For this review, take the finished solid that the model builds, in its own axes (mm). A direction names the side the tool comes from. Coordinates: 2 decimals unless noted, no trailing zeros. Order: outer loops, then holes, each group sorted by start corner. A loop starts at its lowest first (then second) coordinate and runs counter-clockwise, first axis right, second up. Notation, with made-up numbers: (77, 35) - (102, 35) arc R20 ccw to (102, 40) - close; hole circle Ø7 at (57, -4.75). An arc over 180 degrees is marked (long way). One line per item, written item: value. Start each with the question number.
(1) Mouldability with a two-part tool opening along Z and no side actions: class faces 1 (the cylindrical face through (-2.215, 1.014, -28.199)), 2 (the cylindrical face through (-2.199, 1.014, 2.215)), 3 (the cylindrical face through (7.805, 1.014, -27.487)) as released by +Z, released by -Z, zero draft, split by the parting line, or undercut.
(2) Consider section A-A on z = -21. Write out the cut boundary in (x, y), then the cut area to 3 significant figures.
(3) Consider section C-C on x = 0. Write out the cut boundary in (y, z), then the cut area to 3 significant figures.
(4) Consider section B-B on x = 4. Write out the cut boundary in (y, z), then the cut area to 3 significant figures.
(5) Consider section D-D on y = 0.4. Write out the cut boundary in (x, z).
(6) Clearance check with flat-ended pins moving along their axes: pin 1 (3.5 mm diameter, centred on x = 8, z = 0, fed in from +Y); pin 2 (1.8 mm diameter, centred on x = 0, z = -26, fed in from +Y). State where each tip first meets the part, or that it passes through.
(7) For faces 4 (the cylindrical face through (5.715, 1.014, -23.699)), 5 (the cylindrical face through (10.199, 1.014, 2.215)), list the 3-axis set-ups (+Z, -Z, +X, -X, +Y, -Y) from which the entire face can be reached by the end or side of a thin tool; tool diameter is ignored.
(8) To check wall thickness, follow line 1 along Z through (x, y) = (8, 0.8); line 2 along X through (y, z) = (1.4, -26); line 3 along X through (y, z) = (1.95, -8). State the ranges of each line that lie inside material, in increasing order.
```python
from build123d import *

# Parameters (mm, degrees)
SKETCH1_R           = 1.4
BOSS_EXTRUDE2_DEPTH = 5.5
FILLET2_R           = 1
SKETCH2_R           = 1.5
CUT_EXTRUDE1_DEPTH  = 10
SKETCH3_R           = 36.045042524
CUT_EXTRUDE2_DEPTH  = 0.5
SKETCH4_R           = 41.346922652
CUT_EXTRUDE3_DEPTH  = 1
SKETCH5_R           = 64.87410788
CUT_EXTRUDE4_DEPTH  = 2


with BuildPart() as part:
    # Sketch1 → Boss-Extrude2 (new body)
    with BuildSketch(Plane(origin=(0, 0, 0), x_dir=(1, 0, 0), z_dir=(0, 1, 0))):
        Polygon((4, -2.5), (-2.5, -2.5), (-2.5, 28.5), (10.5, 28.5), (10.5, -2.5), align=None)
        with Locations((8, 26)):
            Circle(SKETCH1_R, mode=Mode.SUBTRACT)
        with Locations((0, 26)):
            Circle(SKETCH1_R, mode=Mode.SUBTRACT)
        with Locations((8, 0)):
            Circle(SKETCH1_R, mode=Mode.SUBTRACT)
        Circle(SKETCH1_R, mode=Mode.SUBTRACT)
        Polygon((4, 2), (2, 2), (2, 24), (6, 24), (6, 2), align=None, mode=Mode.SUBTRACT)
    extrude(amount=BOSS_EXTRUDE2_DEPTH)

    # Fillet2
    fillet2_edges = [part.edges().sort_by_distance(p)[0] for p in [
        (6, 2.75, -24),
        (2, 2.75, -24),
        (2, 2.75, -2),
        (6, 2.75, -2),
        (-2.5, 2.75, 2.5),
        (-2.5, 2.75, -28.5),
        (10.5, 2.75, -28.5),
        (10.5, 2.75, 2.5),
    ]]
    fillet(fillet2_edges, radius=FILLET2_R)

    # Sketch2 → Cut-Extrude1 (cut)
    with BuildSketch(Plane(origin=(0, 5.5, 0), x_dir=(1, 0, 0), z_dir=(0, 1, 0))):
        with Locations((0, 26)):
            Circle(SKETCH2_R)
        with Locations((8, 26)):
            Circle(SKETCH2_R)
        with Locations((8, 0)):
            Circle(SKETCH2_R)
        Circle(SKETCH2_R)
    extrude(amount=-CUT_EXTRUDE1_DEPTH, mode=Mode.SUBTRACT)

    # Sketch3 → Cut-Extrude2 (cut)
    with BuildSketch(Plane(origin=(0, 5.5, 0), x_dir=(1, 0, 0), z_dir=(0, 1, 0))):
        Circle(SKETCH3_R)
    extrude(amount=-CUT_EXTRUDE2_DEPTH, mode=Mode.SUBTRACT)

    # Sketch4 → Cut-Extrude3 (cut)
    with BuildSketch(Plane(origin=(0, 5, 0), x_dir=(1, 0, 0), z_dir=(0, 1, 0))):
        Circle(SKETCH4_R)
    extrude(amount=-CUT_EXTRUDE3_DEPTH, mode=Mode.SUBTRACT)

    # Sketch5 → Cut-Extrude4 (cut)
    with BuildSketch(Plane(origin=(0, 4, 0), x_dir=(1, 0, 0), z_dir=(0, 1, 0))):
        Circle(SKETCH5_R)
    extrude(amount=-CUT_EXTRUDE4_DEPTH, mode=Mode.SUBTRACT)


solid = part.part
```
Geometry check:
1. face 1: released by -Z
1. face 2: released by +Z
1. face 3: undercut
2. outline: (-2.5, 0) - (2, 0) - (2, 2) - (-2.5, 2) - close; (6, 0) - (10.5, 0) - (10.5, 2) - (6, 2) - close
2. area: 18.0 mm^2
3. outline: (0, -28.5) - (2, -28.5) - (2, -27.5) - (0, -27.5) - close; (0, -24.5) - (2, -24.5) - (2, -1.5) - (0, -1.5) - close; (0, 1.5) - (2, 1.5) - (2, 2.5) - (0, 2.5) - close
3. area: 50.0 mm^2
4. outline: (0, -28.5) - (2, -28.5) - (2, -24) - (0, -24) - close; (0, -2) - (2, -2) - (2, 2.5) - (0, 2.5) - close
4. area: 18.0 mm^2
5. outline: (-2.5, -27.5) arc R1 ccw to (-1.5, -28.5) - (9.5, -28.5) arc R1 ccw to (10.5, -27.5) - (10.5, 1.5) arc R1 ccw to (9.5, 2.5) - (-1.5, 2.5) arc R1 ccw to (-2.5, 1.5) - close; hole circle Ø3 at (0, -26); hole circle Ø3 at (0, 0); hole (2, -23) arc R1 ccw to (3, -24) - (5, -24) arc R1 ccw to (6, -23) - (6, -3) arc R1 ccw to (5, -2) - (3, -2) arc R1 ccw to (2, -3) - close; hole circle Ø3 at (8, -26); hole circle Ø3 at (8, 0)
6. pin 1: stops at y = 2
6. pin 2: passes through
7. face 4: +Y, -Y
7. face 5: +Z, +X, +Y, -Y
8. line 1: z = -28.5 to -27.5, -24.5 to -1.5, 1.5 to 2.5
8. line 2: x = -2.5 to -1.5, 1.5 to 6.5, 9.5 to 10.5
8. line 3: x = -2.5 to 2, 6 to 10.5
